Here's how the part is built. I have some questions about the finished solid (model axes, mm). A direction names the side the tool comes from. Round coordinates to 2 decimals unless told otherwise and drop trailing zeros. Write each loop counter-clockwise with the first axis right and the second up, starting at its lowest first coordinate (ties: lowest second). Pieces come first, ordered by that corner, then holes. Notation, with made-up numbers: (20, 26.5) -> (77, 26.5) arc R12 ccw to (77, 39.5) -> close; hole circle Ø10 at (27, 73). An arc over 180 degrees is marked (long way). Answer in a Markdown table with one row per item.
from build123d import *

# Parameters (mm, degrees)
F0_R      = 10.5
F0_R_2    = 1.5
F1_DEPTH  = 4
F6_DEPTH  = 0.2
F5_R      = 1.5
F7_DEPTH  = 9.8
F8_DEPTH  = 18.5
F9_R      = 0.7
F10_DEPTH = 8
F11_R     = 1.5
F12_DEPTH = 3.5
F13_R     = 0.85
F14_DEPTH = 26.001
F15_DEPTH = 0.2


with BuildPart() as f1:
    # F0 (on Top) → F1 (new body)
    with BuildSketch(Plane.XY):
        Circle(F0_R)
        with Locations((0, -6)):
            Circle(F0_R_2, mode=Mode.SUBTRACT)
        with Locations((-6.4, 0)):
            Circle(F0_R_2, mode=Mode.SUBTRACT)
        Circle(F0_R_2, mode=Mode.SUBTRACT)
        with Locations((0, 6)):
            Circle(F0_R_2, mode=Mode.SUBTRACT)
    extrude(amount=F1_DEPTH)

    # F2 (on Right) → F3 (revolve, cut)
    with BuildSketch(Plane.YZ):
        with BuildLine():
            Line((-7.5, 0), (-7.5, 2.6428932188))
            ThreePointArc((-7.5, 2.6428932188), (-7.5380602337, 2.4515515026), (-7.6464466094, 2.2893398282))
            Line((-7.6464466094, 2.2893398282), (-8.25, 1.6857864376))
            Line((-8.25, 1.6857864376), (-8.25, 0))
            Line((-8.25, 0), (-7.5, 0))
        make_face()
        with BuildLine():
            Line((-8.65, 4), (-7.6464466094, 2.9964466094))
            ThreePointArc((-7.6464466094, 2.9964466094), (-7.5380602337, 2.834234935), (-7.5, 2.6428932188))
            Line((-7.5, 2.6428932188), (-7.5, 4))
            Line((-7.5, 4), (-8.65, 4))
        make_face()
    revolve(axis=Axis((0, -6, 2), (0, 0, -1)), mode=Mode.SUBTRACT)

    # F2 (on Right) → F4 (revolve, cut)
    with BuildSketch(Plane.YZ):
        with BuildLine():
            Line((7.6464466094, 2.9964466094), (8.65, 4))
            Line((8.65, 4), (7.5, 4))
            Line((7.5, 4), (7.5, 2.6428932188))
            ThreePointArc((7.5, 2.6428932188), (7.5380602337, 2.834234935), (7.6464466094, 2.9964466094))
        make_face()
        with BuildLine():
            ThreePointArc((7.6464466094, 2.2893398282), (7.5380602337, 2.4515515026), (7.5, 2.6428932188))
            Line((7.5, 2.6428932188), (7.5, 0))
            Line((7.5, 0), (8.25, 0))
            Line((8.25, 0), (8.25, 1.6857864376))
            Line((8.25, 1.6857864376), (7.6464466094, 2.2893398282))
        make_face()
    revolve(axis=Axis((0, 6, 2), (0, 0, -1)), mode=Mode.SUBTRACT)

    # F5 (on face) → F6 (join)
    with BuildSketch(Plane.XY.offset(4)):
        with BuildLine():
            Line((-9.5323371892, 4.4027886289), (-2.6806273948, 10.1520557903))
            ThreePointArc((-2.6806273948, 10.1520557903), (-6.7492699017, 8.0434666527), (-9.5323371892, 4.4027886289))
        make_face()
        with BuildLine():
            ThreePointArc((-7.4516245177, -7.3975193172), (-3.5912115049, -9.8667725183), (0.9532417945, -10.4566404778))
            Line((0.9532417945, -10.4566404778), (-7.4516245177, -7.3975193172))
        make_face()
    extrude(amount=F6_DEPTH)

    # F5 (on face) → F7 (join)
    with BuildSketch(Plane.XY.offset(4)):
        with BuildLine():
            ThreePointArc((5.4897887319, -4.658564122), (7.0906158217, 1.2502668792), (3.5653911923, 6.2552366578))
            Line((3.5653911923, 6.2552366578), (2.9914480943, 5.7736412159))
            ThreePointArc((2.9914480943, 5.7736412159), (1.9283628291, 3.7018666706), (-0.2965396247, 3.0146919337))
            Line((-0.2965396247, 3.0146919337), (-4.9240387651, -0.8682408883))
            Line((-4.9240387651, -0.8682408883), (5.4897887319, -4.658564122))
        make_face()
        Circle(F5_R, mode=Mode.SUBTRACT)
    extrude(amount=F7_DEPTH)

    # F5 (on face) → F8 (join)
    with BuildSketch(Plane.XY.offset(4)):
        with BuildLine():
            ThreePointArc((7.4648121374, -5.3774138536), (9.0602313277, 1.5975632345), (5.1754450242, 7.6062322343))
            Line((5.1754450242, 7.6062322343), (3.5653911923, 6.2552366578))
            ThreePointArc((3.5653911923, 6.2552366578), (7.0906158217, 1.2502668792), (5.4897887319, -4.658564122))
            Line((5.4897887319, -4.658564122), (7.4648121374, -5.3774138536))
        make_face()
    extrude(amount=F8_DEPTH)

    # F9 (on face) → F10 (cut)
    with BuildSketch(Plane.XY.offset(22.5)):
        with Locations((5.2113912337, 6.3309873961)):
            Circle(F9_R)
        with Locations((8.0754235747, 1.4239150569)):
            Circle(F9_R)
        with Locations((7.3951047667, -3.5429402323)):
            Circle(F9_R)
    extrude(amount=-F10_DEPTH, mode=Mode.SUBTRACT)

    # F11 (on face) → F12 (join)
    with BuildSketch(Plane(origin=(0, 0, 0), x_dir=(1, 0, 0), z_dir=(0, 0, -1))):
        with BuildLine():
            ThreePointArc((-6.7538286642, 6.24706318), (-9.1873917197, -0.4814907974), (-6.0638345699, -6.9188084457))
            Line((-6.0638345699, -6.9188084457), (4.9931476738, 0.2616797812))
            Line((4.9931476738, 0.2616797812), (-6.7538286642, 6.24706318))
        make_face()
        with Locations((-6.4, 0)):
            Circle(F11_R, mode=Mode.SUBTRACT)
        Circle(F11_R, mode=Mode.SUBTRACT)
    extrude(amount=F12_DEPTH)

    # F13 (on face) → F14 (cut, through all)
    with BuildSketch(Plane(origin=(0, 0, -3.5), x_dir=(1, 0, 0), z_dir=(0, 0, -1))):
        with Locations((-5.9440995908, -5.6486883482)):
            Circle(F13_R)
        with Locations((-6.5019859038, 4.9964166467)):
            Circle(F13_R)
    extrude(amount=-F14_DEPTH, mode=Mode.SUBTRACT)

    # F11 (on face) → F15 (join)
    with BuildSketch(Plane(origin=(0, 0, 0), x_dir=(1, 0, 0), z_dir=(0, 0, -1))):
        with BuildLine():
            Line((8.924719634, -5.5316705845), (1.4234220313, -10.4030702065))
            ThreePointArc((1.4234220313, -10.4030702065), (5.7187098677, -8.8060409634), (8.924719634, -5.5316705845))
        make_face()
        with BuildLine():
            ThreePointArc((8.2976120605, 6.4342547427), (4.7669002473, 9.355568504), (0.3282074346, 10.4948692169))
            Line((0.3282074346, 10.4948692169), (8.2976120605, 6.4342547427))
        make_face()
    extrude(amount=F15_DEPTH)


solid = f1.part
1) I want a section at B-B, the plane x = -6.4. List the corners of the cut face in (y, z) for me.
Response:
| item | result |
|---|---|
| outline | (-8.32, 0) -> (-6.07, 0) -> (-6.07, -3.5) -> (-5.84, -3.5) -> (-5.84, 4) -> (-7.78, 4) -> (-7.78, 4.2) -> (-8.32, 4.2) -> close; (-4.15, -3.5) -> (-1.5, -3.5) -> (-1.5, 4) -> (-4.15, 4) -> close; (1.5, -3.5) -> (4.93, -3.5) -> (4.93, 4) -> (1.5, 4) -> close; (6.37, -3.5) -> (6.61, -3.5) -> (6.61, 0) -> (8.32, 0) -> (8.32, 4.2) -> (7.03, 4.2) -> (7.03, 4) -> (6.37, 4) -> close |
2) We'd pull the mould along X, two halves only. Please class faces 1 (the face through (5, 6, 14.5)), 2 (the face through (7.075, 1.337, 18.089)), 3 (the face through (9.078, 1.496, 13.12)), 4 (the face through (-6, 8, 4.2)): +X half, -X half, draft (parallel to the pull), parting line (faces both ways), or undercut.
Response:
| item | result |
|---|---|
| face 1 | undercut |
| face 2 | -X half |
| face 3 | +X half |
| face 4 | draft |
3) For pin 1 (1.5 mm diameter, centred on x = -1, z = 15, fed in from -Y); pin 2 (2 mm diameter, centred on x = 6, y = -8, fed in from -Z); pin 3 (1.1 mm diameter, centred on x = 8.08, y = 1.42, fed in from +Z); pin 4 (3.5 mm diameter, centred on x = -3, y = -9.5, fed in from +Z), each with a flat end and sliding along its axis, tell me the tip position at first contact or that it passes through.
Response:
| item | result |
|---|---|
| pin 1 | passes through |
| pin 2 | stops at z = -0.2 |
| pin 3 | stops at z = 14.5 |
| pin 4 | stops at z = 4.2 |
4) I need wall thicknesses on line 1 (X direction, y = 0, z = 2); line 2 (Y direction, x = -0.25, z = 1.5); line 3 (Y direction, x = 5.75, z = 17.25). Which ranges of each line are inside material? Lowest first, please. Write a range as [from, to].
Response:
| item | result |
|---|---|
| line 1 | x = [-10.5, -7.9], [-4.9, -1.5], [1.5, 10.5] |
| line 2 | y = [-10.5, -8.24], [-3.76, -1.48], [1.48, 3.76], [8.24, 10.5] |
| line 3 | y = [-4.75, -4.33], [4.33, 5.88], [6.78, 7.18] |
5) Which directions (+Z, -Z, +X, -X, +Y, -Y) give clear straight access to the entire face, cutting with the end or side of a thin tool? Please do faces 5 (the face through (7.4, 0.2, 22.5)), 6 (the face through (7.52, 1, 18.56)), 7 (the face through (2, -2, 0)), 8 (the face through (5, -9, -0.2)), 9 (the face through (-5.014, 0.575, 0.303)).
Response:
| item | result |
|---|---|
| face 5 | +Z, +X, -X, +Y, -Y |
| face 6 | +Z |
| face 7 | -Z |
| face 8 | -Z, +X, -X, -Y |
| face 9 | +Z, -Z |
6) I want a section at C-C, the plane z = 18. List the corners of the cut face in (x, y) for me, and give its area (3 significant figures).
Response:
| item | result |
|---|---|
| outline | (3.57, 6.26) arc R7.2 cw to (5.49, -4.66) -> (7.46, -5.38) arc R9.2 ccw to (5.18, 7.61) -> close; hole circle Ø1.4 at (5.21, 6.33); hole circle Ø1.4 at (7.4, -3.54); hole circle Ø1.4 at (8.08, 1.42) |
| area | 22.7 mm^2 |
7) I want a section at A-A, the plane z = 6. List the corners of the cut face in (x, y) for me.
Response:
| item | result |
|---|---|
| outline | (-4.92, -0.87) -> (7.46, -5.38) arc R9.2 ccw to (5.18, 7.61) -> (2.99, 5.77) arc R3 cw to (-0.3, 3.01) -> close; hole circle Ø3 at (0, 0) |
